The listing builds one solid part. Answer for the finished solid, in the listing's coordinates (mm). Coordinates: 2 decimals unless noted, no trailing zeros. Order: outer loops, then holes, each group sorted by start corner. A loop starts at its lowest first (then second) coordinate and runs counter-clockwise, first axis right, second up. Notation, with made-up numbers: M -36,4 L 1,4 A17 cw 1,36 Z; hole C 25.5,-7 d6. An arc over 180 degrees is marked long. One line per item, written item: value. Start each with the question number.
Q1. Each of these flat-tipped pins is pushed along its axis until it touches: pin 1 Ø2 at (x, z) = (-9.5, 2.5) entering from +Y; pin 2 Ø1 at (x, z) = (6, 5.5) entering from -Y; pin 3 Ø1 at (x, z) = (-5.5, 6) entering from +Y. Where does it stop, or does it pass through?
Q2. Determine the mould class of faces 1 (the cylindrical face through (-10.49, -142.15, 3.94)), 2 (the cylindrical face through (0, 128, 4)), 3 (the cylindrical face through (-10.65, 141.99, 3.94)) for opening direction Y: pulls with the +Y half, pulls with the -Y half, needs draft (parallel to the pull), parting line crosses it, or undercut.
Q3. The part is cut by section B-B on y = 125. Give the vertices of the cut face in (x, z).
Q4. The part is cut by section A-A on x = 0. Give the vertices of the cut face in (y, z).
Q5. Straight lines are drawn through the part: line 1 along Y through (x, z) = (0, 5.75); line 2 along Y through (x, z) = (4.25, 7.75); line 3 along Y through (x, z) = (-4.5, 2.5). For each, find the intervals that lie inside material, in ascending order. Write a range as [from, to].
```python
from build123d import *

# Parameters (mm, degrees)
SKETCH1_R           = 3
BOSS_EXTRUDE1_DEPTH = 8


with BuildPart() as part:
    # Sketch1 → Boss-Extrude1 (new body)
    with BuildSketch(Plane.XY):
        with BuildLine():
            ThreePointArc((3.5, 145), (10.571067812, 142.071067812), (13.5, 135))
            Line((13.5, 135), (13.5, -135))
            ThreePointArc((13.5, -135), (10.571067812, -142.071067812), (3.5, -145))
            Line((3.5, -145), (-3.5, -145))
            ThreePointArc((-3.5, -145), (-10.571067812, -142.071067812), (-13.5, -135))
            Line((-13.5, -135), (-13.5, 135))
            ThreePointArc((-13.5, 135), (-10.571067812, 142.071067812), (-3.5, 145))
            Line((-3.5, 145), (3.5, 145))
        make_face()
        with Locations((0, 125)):
            Circle(SKETCH1_R, mode=Mode.SUBTRACT)
    extrude(amount=BOSS_EXTRUDE1_DEPTH)


solid = part.part
```
Output:
1. pin 1: stops at y = 143.66
1. pin 2: stops at y = -144.8
1. pin 3: stops at y = 144.89
2. face 1: pulls with the -Y half
2. face 2: undercut
2. face 3: pulls with the +Y half
3. outline: M -13.5,0 L -3,0 L -3,8 L -13.5,8 Z; M 3,0 L 13.5,0 L 13.5,8 L 3,8 Z
4. outline: M -145,0 L 122,0 L 122,8 L -145,8 Z; M 128,0 L 145,0 L 145,8 L 128,8 Z
5. line 1: y = [-145, 122], [128, 145]
5. line 2: y = [-144.97, 144.97]
5. line 3: y = [-144.95, 144.95]
